Design review of the part built by this model. Coordinates are the model's own, in mm. Give positions to 0.01 mm unless a question says otherwise; leave off trailing zeros. Write each loop counter-clockwise with the first axis right and the second up, starting at its lowest first coordinate (ties: lowest second). Pieces come first, ordered by that corner, then holes. Notation, with made-up numbers: (-18, 39) -> (40, 39) arc R18 cw to (40, 47) -> close; hole circle Ø11 at (85.25, -38). An arc over 180 degrees is marked (long way). Answer as a JSON object with one key per item and string values.
```python
from build123d import *

# Parameters (mm, degrees)
BOSS_EXTRUDE1_DEPTH     = 37.5
CUT_EXTRUDE1_DEPTH      = 39.810570802
CUT_EXTRUDE1_DEPTH_BACK = 39.810570802
SKETCH2_R               = 3
FILLET1_R               = 1


with BuildPart() as part:
    # Sketch1 → Boss-Extrude1 (new, symmetric)
    with BuildSketch(Plane(origin=(0, 0, 0), x_dir=(1, 0, 0), z_dir=(0, 1, 0))):
        with BuildLine():
            Line((-6, 7.350239011), (-6, -7.350239011))
            ThreePointArc((-6, -7.350239011), (0, -8.000650348), (6, -7.350239011))
            Line((6, -7.350239011), (6, 7.350239011))
            ThreePointArc((6, 7.350239011), (0, 5.999349652), (-6, 7.350239011))
        make_face()
    extrude(amount=BOSS_EXTRUDE1_DEPTH, both=True)

    # Sketch2 → Cut-Extrude1 (cut, two sides: drawn at the far end of the back side and taken through both)
    with BuildSketch(Plane(origin=(0, 0, 0), x_dir=(0, 0, -1), z_dir=(1, 0, 0)).offset(-CUT_EXTRUDE1_DEPTH_BACK)):
        with Locations((0, 30)):
            Circle(SKETCH2_R)
        with Locations((0, -30)):
            Circle(SKETCH2_R)
    extrude(amount=CUT_EXTRUDE1_DEPTH + CUT_EXTRUDE1_DEPTH_BACK, mode=Mode.SUBTRACT)

    # Fillet1
    fillet1_edges = [part.edges().sort_by_distance(p)[0] for p in [
        (0, 37.5, 8.000650348),
        (6, 37.5, 0),
        (0, 37.5, -5.999349652),
        (0, -37.5, 8.000650348),
        (0, -37.5, -5.999349652),
        (6, 0, -7.350239011),
        (6, 0, 7.350239011),
        (-6, 0, 7.350239011),
        (-6, 0, -7.350239011),
        (-6, 37.5, 0),
    ]]
    fillet(fillet1_edges, radius=FILLET1_R)


solid = part.part
```
(1) For line 1 along Y through (x, z) = (2, 0); line 2 along Z through (x, y) = (0, 30); line 3 along Z through (x, y) = (3, 30), list the stretches that pass through material, from the lowest coordinate up.
Here are the results:
{"line 1": "y = -37.5 to -33, -27 to 27, 33 to 37.5", "line 2": "z = -6 to -3, 3 to 8", "line 3": "z = -6.32 to -3, 3 to 7.84"}
(2) We need section C-C, the plane y = 24. State the section outline as (x, z) points, then the cut area to 3 significant figures.
Here are the results:
{"outline": "(-6, -5.86) arc R1 ccw to (-4.67, -6.8) arc R14 cw to (4.67, -6.8) arc R1 ccw to (6, -5.86) -> (6, 6.53) arc R1 ccw to (5.19, 7.52) arc R28 ccw to (-5.19, 7.52) arc R1 ccw to (-6, 6.53) -> close", "area": "169 mm²"}
(3) We need section D-D, the plane x = 2. Give the number of separate pieces and of enclosed holes in the cut face, then the cut area to 3 significant figures.
Here are the results:
{"separate pieces": "1", "enclosed holes": "2", "area": "998 mm²"}
(4) We need section B-B, the plane z = 0. State the section outline as (x, y) points.
Here are the results:
{"outline": "(-6, -37.5) -> (6, -37.5) -> (6, -33) -> (-6, -33) -> close; (-6, -27) -> (6, -27) -> (6, 27) -> (-6, 27) -> close; (-6, 33) -> (6, 33) -> (6, 36.5) arc R1 ccw to (5, 37.5) -> (-5, 37.5) arc R1 ccw to (-6, 36.5) -> close"}
(5) The part is to be moulded in two halves that separate along Z. For faces 1 (the flat face through (6, 0, 0)), 2 (the cylindrical face through (-0.08, 32.03, 2.21)), 3 (the cylindrical face through (-0.08, -32.93, 0.65)), 4 (the cylindrical face through (-5.588, -1.018, -6.666)), say which applies: +Z half, -Z half, draft (parallel to the pull), parting line (faces both ways), or undercut.
Here are the results:
{"face 1": "draft", "face 2": "undercut", "face 3": "undercut", "face 4": "-Z half"}
(6) We need section A-A, the plane y = -30. State the section outline as (x, z) points, then the cut area to 3 significant figures.
Here are the results:
{"outline": "(-6, -5.86) arc R1 ccw to (-4.67, -6.8) arc R14 cw to (4.67, -6.8) arc R1 ccw to (6, -5.86) -> (6, -3) -> (-6, -3) -> close; (-6, 3) -> (6, 3) -> (6, 6.53) arc R1 ccw to (5.19, 7.52) arc R28 ccw to (-5.19, 7.52) arc R1 ccw to (-6, 6.53) -> close", "area": "97.5 mm²"}
(7) Clearance check with a flat-ended pin moving along its axis: pin 1 (1.5 mm diameter, centred on x = 2.5, y = 30, fed in from +Z). State where the tip first meets the part, or that it passes through.
Here are the results:
{"pin 1": "stops at z = 7.95"}
